```python
from build123d import *

# Parameters (mm, degrees)
SKETCH1_W           = 68
SKETCH1_H           = 34.5
BOSS_EXTRUDE1_DEPTH = 2
SKETCH2_R           = 1.45
BOSS_EXTRUDE2_DEPTH = 2
SKETCH3_R           = 1.5
CUT_EXTRUDE1_DEPTH  = 39.17803688


with BuildPart() as part:
    # Sketch1 → Boss-Extrude1 (new body)
    with BuildSketch(Plane.XY):
        Rectangle(SKETCH1_W, SKETCH1_H)
    extrude(amount=BOSS_EXTRUDE1_DEPTH)

    # Sketch2 → Boss-Extrude2 (add)
    with BuildSketch(Plane.XY.offset(2)):
        with Locations(Location((-7.25, 0, 0), (0, 0, 180))):
            Circle(SKETCH2_R)
        with Locations(Location((7.25, 0, 0), (0, 0, 180))):
            Circle(SKETCH2_R)
    extrude(amount=BOSS_EXTRUDE2_DEPTH)

    # Sketch3 → Cut-Extrude1 (cut, through all)
    with BuildSketch(Plane.XY.offset(2)):
        Circle(SKETCH3_R)
    extrude(amount=-CUT_EXTRUDE1_DEPTH, mode=Mode.SUBTRACT)


solid = part.part
```
Part model, mm, in its own coordinate system. A direction names the side the tool comes from. Give positions to 0.01 mm unless a question says otherwise; leave off trailing zeros. Order: outer loops, then holes, each group sorted by start corner. A loop starts at its lowest first (then second) coordinate and runs counter-clockwise, first axis right, second up. Notation, with made-up numbers: M 77,45.5 L 111,45.5 A7 ccw 111,49.5 Z; hole C -30.75,89.25 d3. An arc over 180 degrees is marked long. Use a Markdown table: item, result. Add a question column.
(1) Saw through at D-D, the plane x = 7.25. Give the cut face in (y, z).
(2) Drop flat-ended pins along their axis: P1, Ø2.5, axis at x = 0, y = 0, coming from the -Z side; P2, Ø2, axis at x = -11, y = -1, coming from the +Z side. Give the stop position or say it passes through.
(3) Mould opens along X. For faces 1 (the face through (-1.5, 0.07, 1.01)), 2 (the face through (-34, 0, 1)), 3 (the face through (7, 0, 4)) say: +X half, -X half, draft (parallel to the pull), parting line (faces both ways), or undercut.
(4) Saw through at A-A, the plane y = 0. Give the cut face in (x, z).
(5) Probe line 1 along Y through (x, z) = (0, 1.2); line 2 along Z through (x, y) = (21, 5); line 3 along Y through (x, z) = (6, 3.5). List the from-to ranges inside material, lowest first. Write a range as [from, to].
(6) 3-axis set-ups, long thin cutter, end or side, ignore diameter. For faces 4 (the face through (8.7, -0.06, 2.99)), 5 (the face through (-7, 0, 4)): which of +Z, -Z, +X, -X, +Y, -Y reach the whole face in a straight line?
(7) Saw through at B-B, the plane x = 0. Give the cut face in (y, z).
(8) Saw through at C-C, the plane z = 3.4. Give the cut face in (x, y).
Answer key:
| question | item | result |
|---|---|---|
| 1 | outline | M -17.25,0 L 17.25,0 L 17.25,2 L 1.45,2 L 1.45,4 L -1.45,4 L -1.45,2 L -17.25,2 Z |
| 2 | P1 | through |
| 2 | P2 | z = 2 |
| 3 | face 1 | undercut |
| 3 | face 2 | -X half |
| 3 | face 3 | draft |
| 4 | outline | M -34,0 L -1.5,0 L -1.5,2 L -5.8,2 L -5.8,4 L -8.7,4 L -8.7,2 L -34,2 Z; M 1.5,0 L 34,0 L 34,2 L 8.7,2 L 8.7,4 L 5.8,4 L 5.8,2 L 1.5,2 Z |
| 5 | line 1 | [-17.25, -1.5], [1.5, 17.25] |
| 5 | line 2 | [0, 2] |
| 5 | line 3 | [-0.73, 0.73] |
| 6 | face 4 | +Z |
| 6 | face 5 | +Z, +X, -X, +Y, -Y |
| 7 | outline | M -17.25,0 L -1.5,0 L -1.5,2 L -17.25,2 Z; M 1.5,0 L 17.25,0 L 17.25,2 L 1.5,2 Z |
| 8 | outline | C -7.25,0 d2.9; C 7.25,0 d2.9 |
